Geometry check sheet. Reference: the model listing, model coordinates, mm. Face numbers are marked on the shaded views. A direction names the side the tool comes from. Round coordinates to 2 decimals unless told otherwise and drop trailing zeros. Loops run counter-clockwise (first coordinate to the right, second up) from the corner with the lowest first, then second, coordinate; pieces in that order, holes last. Notation, with made-up numbers: (73.5, -37) - (132.5, -37) arc R35 cw to (132.5, -4) - close; hole circle Ø11 at (1, 5). An arc over 180 degrees is marked (long way). Write item = value, one per line.
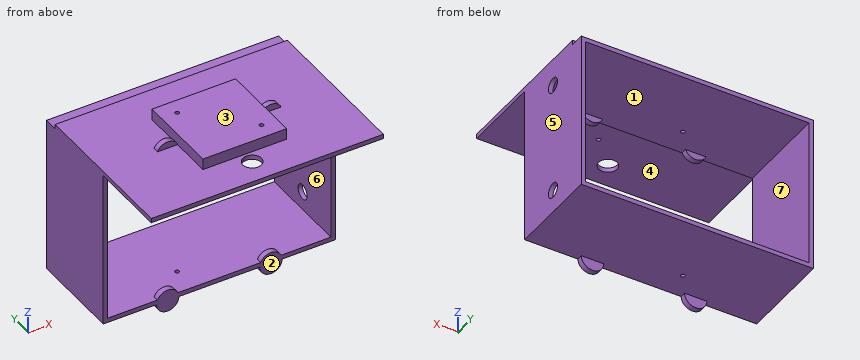
```python
from build123d import *

# Parameters (mm, degrees)
SKETCH1_W           = 124.8
SKETCH1_H           = 84.8
SKETCH1_W_2         = 120
SKETCH1_H_2         = 80
BOSS_EXTRUDE1_DEPTH = 50
SKETCH2_W           = 124.8
SKETCH2_H           = 84.8
BOSS_EXTRUDE2_DEPTH = 2.4
SKETCH3_W           = 45
SKETCH3_H           = 45
BOSS_EXTRUDE3_DEPTH = 6
SKETCH4_R           = 1.1
SKETCH4_R_2         = 5
CUT_EXTRUDE1_DEPTH  = 123.800651464
SKETCH5_R           = 4
CUT_EXTRUDE2_DEPTH  = 3
SKETCH6_R           = 6
BOSS_EXTRUDE4_DEPTH = 3


with BuildPart() as part:
    # Sketch1 → Boss-Extrude1 (new body)
    with BuildSketch(Plane(origin=(0, 0, 0), x_dir=(1, 0, 0), z_dir=(0, 1, 0))):
        Rectangle(SKETCH1_W, SKETCH1_H)
        Rectangle(SKETCH1_W_2, SKETCH1_H_2, mode=Mode.SUBTRACT)
    extrude(amount=BOSS_EXTRUDE1_DEPTH)

    # Sketch2 → Boss-Extrude2 (add)
    with BuildSketch(Plane.XY.offset(42.4)):
        Rectangle(SKETCH2_W, SKETCH2_H)
    extrude(amount=BOSS_EXTRUDE2_DEPTH)

    # Sketch3 → Boss-Extrude3 (add)
    with BuildSketch(Plane.XY.offset(44.8)):
        Rectangle(SKETCH3_W, SKETCH3_H)
    extrude(amount=BOSS_EXTRUDE3_DEPTH)

    # Sketch4 → Cut-Extrude1 (cut, through all)
    with BuildSketch(Plane.XY.offset(50.8)):
        with Locations((-14.1, 14.1)):
            Circle(SKETCH4_R)
        with Locations((14.1, -14.1)):
            Circle(SKETCH4_R)
        with Locations(Location((0, -29, 0), (0, 0, 180))):
            Circle(SKETCH4_R_2)
    extrude(amount=-CUT_EXTRUDE1_DEPTH, mode=Mode.SUBTRACT)

    # Sketch5 → Cut-Extrude2 (cut)
    with BuildSketch(Plane(origin=(62.4, 0, 0), x_dir=(0, 0, -1), z_dir=(1, 0, 0))):
        with Locations((-30, 25)):
            Circle(SKETCH5_R)
        with Locations((30, 25)):
            Circle(SKETCH5_R)
    extrude(amount=-CUT_EXTRUDE2_DEPTH, mode=Mode.SUBTRACT)

    # Sketch6 → Boss-Extrude4 (add)
    with BuildSketch(Plane(origin=(0, 0, 0), x_dir=(1, 0, 0), z_dir=(0, 1, 0))):
        with Locations((-27.75, -42.4)):
            Circle(SKETCH6_R)
        with Locations((27.75, -42.4)):
            Circle(SKETCH6_R)
        with Locations((-27.75, 42.4)):
            Circle(SKETCH6_R)
        with Locations((27.75, 42.4)):
            Circle(SKETCH6_R)
    extrude(amount=BOSS_EXTRUDE4_DEPTH)


solid = part.part
```
(1) Scan lines: L1, parallel to X at y = 46, z = -1.5; L2, parallel to Y at x = -14.1, z = 47; L3, parallel to Y at x = 61.6, z = 30. Record each from-to range of solid material in increasing order. Write a range as [from, to].
Answers follow:
L1 = [-62.4, -60], [60, 62.4]
L2 = [-22.5, 13], [15.2, 22.5]
L3 = [0, 21], [29, 50]
(2) Set-up check for the marked faces 1, 2 and 3: record each of +Z, -Z, +X, -X, +Y, -Y from which the full face is reachable in a straight line by a thin tool's end or side.
Answers follow:
face_1 = +Y
face_2 = -Z, +X, -X, -Y
face_3 = +Z, +X, -X, +Y, -Y
(3) Gauge pin test, flat ends, axial feed: pin 1 (3 mm diameter, centred on x = 29.5, z = -45.5, fed in from +Y); pin 2 (1 mm diameter, centred on x = -47, y = 37.5, fed in from -Z); pin 3 (3 mm diameter, centred on x = 1.5, z = 47, fed in from +Y). Record the tip position at first contact, or that the pin passes through.
Answers follow:
pin_1 = 3
pin_2 = -42.4
pin_3 = 22.5
(4) Section check D-D (x = 27.75). Enter the section's corners in (y, z).
Answers follow:
outline = (-42.4, 42.4) - (0, 42.4) - (0, 36.4) - (3, 36.4) - (3, 40) - (50, 40) - (50, 42.4) - (42.4, 42.4) - (42.4, 44.8) - (3, 44.8) - (3, 48.4) - (0, 48.4) - (0, 44.8) - (-42.4, 44.8) - close; (0, -48.4) - (3, -48.4) - (3, -42.4) - (50, -42.4) - (50, -40) - (3, -40) - (3, -36.4) - (0, -36.4) - close
(5) Section check C-C (y = 32.5). Enter the section's corners in (x, z), then the cut area to 3 significant figures.
Answers follow:
outline = (-62.4, -42.4) - (62.4, -42.4) - (62.4, 44.8) - (-62.4, 44.8) - close; hole (-60, -40) - (60, -40) - (60, 40) - (-60, 40) - close
area = 1,280 mm²
(6) Section check B-B (z = -17.5). Enter the section's corners in (x, y), then the cut area to 3 significant figures.
Answers follow:
outline = (-62.4, 0) - (-60, 0) - (-60, 50) - (-62.4, 50) - close; (60, 0) - (62.4, 0) - (62.4, 50) - (60, 50) - close
area = 240 mm²
(7) Mould release check, pull along Z, two halves, no side actions. Record for the marked faces 4, 5, 6 and 7: pulls with the +Z half, pulls with the -Z half, needs draft (parallel to the pull), parting line crosses it, or undercut.
Answers follow:
face_4 = pulls with the -Z half
face_5 = needs draft
face_6 = undercut
face_7 = undercut
(8) Section check A-A (x = 42.5). Enter the section's corners in (y, z).
Answers follow:
outline = (-42.4, 42.4) - (0, 42.4) - (0, 40) - (50, 40) - (50, 42.4) - (42.4, 42.4) - (42.4, 44.8) - (-42.4, 44.8) - close; (0, -42.4) - (50, -42.4) - (50, -40) - (0, -40) - close
